Work out the finished part from the listing and answer in its coordinate system (mm). Round coordinates to 2 decimals unless told otherwise and drop trailing zeros. Order: outer loops, then holes, each group sorted by start corner. A loop starts at its lowest first (then second) coordinate and runs counter-clockwise, first axis right, second up. Notation, with made-up numbers: (-16, -6) - (6, -6) arc R32 cw to (6, 31) - close; hole circle Ø6 at (-25, -23). An arc over 180 degrees is marked (long way). Answer in a Markdown table with one row per item.
from build123d import *

# Parameters (mm, degrees)
SKETCH1_R                                        = 3.5
BODY_DEPTH                                       = 3.175
F_6_GIMBAL_CLEARANCE_HOLE_D                      = 3.7973
F_6_GIMBAL_CLEARANCE_HOLE_DEPTH                  = 12
F_6_GIMBAL_CLEARANCE_HOLE_TIP                    = 1.140824014
CSK_FOR_M2_5_FLAT_HEAD_MACHINE_SCREW_D           = 2.9
CSK_FOR_M2_5_FLAT_HEAD_MACHINE_SCREW_CSINK_D     = 5.5
CSK_FOR_M2_5_FLAT_HEAD_MACHINE_SCREW_CSINK_ANGLE = 90
F_6_CIRCULAR_CLEARANCE_HOLES_D                   = 3.7973
F_6_CIRCULAR_CLEARANCE_HOLES_DEPTH               = 12
F_6_CIRCULAR_CLEARANCE_HOLES_TIP                 = 1.140824014
MOTOR_START                                      = 1.82626
SKETCH1_3_R                                      = 5
MOTOR_COLLAR_RELIEF_DEPTH                        = 135.039371942
F_6_32_TAPPED_HOLE_D                             = 2.7051
F_6_32_TAPPED_HOLE_DEPTH                         = 180.4416
F_6_32_TAPPED_HOLE_TIP                           = 0.81269403
FILLET1_R                                        = 6.35


with BuildPart() as part:
    # Sketch1 → Body (new body)
    with BuildSketch(Plane.XY):
        with BuildLine():
            Line((-29.36875, 100.140279829), (-29.36875, 87.440279829))
            Line((-29.36875, 87.440279829), (0, 87.440279829))
            Line((0, 87.440279829), (19.184718186, 66.158495963))
            Line((19.184718186, 66.158495963), (39.064677756, 56.735799561))
            Line((39.064677756, 56.735799561), (54.483635505, 89.266642494))
            ThreePointArc((54.483635505, 89.266642494), (49.996218262, 103.531501135), (35.431784746, 100.140279829))
            Line((35.431784746, 100.140279829), (6.35, 100.140279829))
            Line((6.35, 100.140279829), (6.35, 117.602779829))
            ThreePointArc((6.35, 117.602779829), (0, 123.952779829), (-6.35, 117.602779829))
            Line((-6.35, 117.602779829), (-6.35, 100.140279829))
            Line((-6.35, 100.140279829), (-29.36875, 100.140279829))
        make_face()
        with Locations((44.54365572, 93.977990695)):
            Circle(SKETCH1_R, mode=Mode.SUBTRACT)
    extrude(amount=BODY_DEPTH)

    # #6 Gimbal Clearance Hole
    with Locations(Plane(origin=(0, 108.077779829, 0), x_dir=(-1, 0, 0), z_dir=(0, 0, -1))):
        with Locations((0, 0), (0, 11.1125)):
            Hole(F_6_GIMBAL_CLEARANCE_HOLE_D / 2, depth=F_6_GIMBAL_CLEARANCE_HOLE_DEPTH)
            with Locations((0, 0, -(F_6_GIMBAL_CLEARANCE_HOLE_DEPTH + F_6_GIMBAL_CLEARANCE_HOLE_TIP / 2))):  # 118° drill point
                Cone(0, F_6_GIMBAL_CLEARANCE_HOLE_D / 2, F_6_GIMBAL_CLEARANCE_HOLE_TIP, mode=Mode.SUBTRACT)

    # CSK for M2.5 Flat Head Machine Screw (through all)
    with Locations(Plane(origin=(50.605833546, 97.477990695, 0), x_dir=(-1, 0, 0), z_dir=(0, 0, -1))):
        with Locations((0, 0), (6.062177826, -10.5), (12.124355653, 0)):
            CounterSinkHole(CSK_FOR_M2_5_FLAT_HEAD_MACHINE_SCREW_D / 2, CSK_FOR_M2_5_FLAT_HEAD_MACHINE_SCREW_CSINK_D / 2, counter_sink_angle=CSK_FOR_M2_5_FLAT_HEAD_MACHINE_SCREW_CSINK_ANGLE)

    # #6 Circular Clearance Holes
    with Locations(Plane(origin=(-20.32, 93.790279829, 0), x_dir=(-1, 0, 0), z_dir=(0, 0, -1))):
        with Locations((0, 0), (-20.32, 0), (-40.64, 0)):
            Hole(F_6_CIRCULAR_CLEARANCE_HOLES_D / 2, depth=F_6_CIRCULAR_CLEARANCE_HOLES_DEPTH)
            with Locations((0, 0, -(F_6_CIRCULAR_CLEARANCE_HOLES_DEPTH + F_6_CIRCULAR_CLEARANCE_HOLES_TIP / 2))):  # 118° drill point
                Cone(0, F_6_CIRCULAR_CLEARANCE_HOLES_D / 2, F_6_CIRCULAR_CLEARANCE_HOLES_TIP, mode=Mode.SUBTRACT)

    # Sketch1<3> → Motor Collar Relief (cut, through all)
    with BuildSketch(Plane.XY.offset(MOTOR_START)):
        with Locations((44.54365572, 93.977990695)):
            Circle(SKETCH1_3_R)
    extrude(amount=MOTOR_COLLAR_RELIEF_DEPTH, mode=Mode.SUBTRACT)

    # #6-32 Tapped Hole
    with Locations(Plane(origin=(32.122828644, 67.772589444, 0), x_dir=(-1, 0, 0), z_dir=(0, 0, -1))):
        with Locations((0, 0)):
            Hole(F_6_32_TAPPED_HOLE_D / 2, depth=F_6_32_TAPPED_HOLE_DEPTH)
            with Locations((0, 0, -(F_6_32_TAPPED_HOLE_DEPTH + F_6_32_TAPPED_HOLE_TIP / 2))):  # 118° drill point
                Cone(0, F_6_32_TAPPED_HOLE_D / 2, F_6_32_TAPPED_HOLE_TIP, mode=Mode.SUBTRACT)

    # Fillet1
    fillet1_edges = [part.edges().sort_by_distance(p)[0] for p in [
        (0, 87.440279829, 1.5875),
        (-29.36875, 87.440279829, 1.5875),
        (-29.36875, 100.140279829, 1.5875),
        (-6.35, 100.140279829, 1.5875),
        (6.35, 100.140279829, 1.5875),
        (35.431784746, 100.140279829, 1.5875),
        (39.064677756, 56.735799561, 1.5875),
        (19.184718186, 66.158495963, 1.5875),
    ]]
    fillet(fillet1_edges, radius=FILLET1_R - 0.0001)  # a hair under: the kernel refuses the full size


solid = part.part
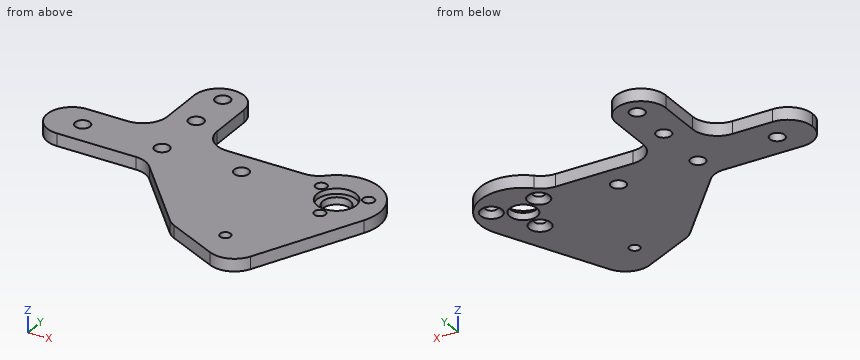
1) Find section D-D, the plane y = 115.5. Give the vertices of the cut face in (x, z) (3 decimals), then the cut area to 3 significant figures.
Filled in:
| item | result |
|---|---|
| outline | (-6.35, 0) - (6.35, 0) - (6.35, 3.175) - (-6.35, 3.175) - close |
| area | 40.3 mm^2 |
2) Find the intervals of material crossed by probe 1 along Y at (x, z) = (20.32, 0.7); probe 2 along Y at (x, z) = (0, 1.45); probe 3 along Y at (x, z) = (-23, 0.6), in increasing order. Write a range as from..to.
Filled in:
| item | result |
|---|---|
| probe 1 | y = 65.62..91.89, 95.69..100.14 |
| probe 2 | y = 86.78..91.89, 95.69..106.18, 109.98..117.29, 121.09..123.95 |
| probe 3 | y = 87.44..100.14 |
3) Find section C-C, the plane x = 0. Give the vertices of the cut face in (y, z) (3 decimals).
Filled in:
| item | result |
|---|---|
| outline | (86.777, 0) - (91.892, 0) - (91.892, 3.175) - (86.777, 3.175) - close; (95.689, 0) - (106.179, 0) - (106.179, 3.175) - (95.689, 3.175) - close; (109.976, 0) - (117.292, 0) - (117.292, 3.175) - (109.976, 3.175) - close; (121.089, 0) - (123.953, 0) - (123.953, 3.175) - (121.089, 3.175) - close |
4) Find section A-A, the plane x = -20.32. Give the vertices of the cut face in (y, z) (3 decimals).
Filled in:
| item | result |
|---|---|
| outline | (87.44, 0) - (91.892, 0) - (91.892, 3.175) - (87.44, 3.175) - close; (95.689, 0) - (100.14, 0) - (100.14, 3.175) - (95.689, 3.175) - close |
5) Each of these flat-tipped pins is pushed along its axis until it touches: pin 1 (4 mm diameter, centred on x = 50.61, y = 97.48, fed in from -Z); pin 2 (2.5 mm diameter, centred on x = 38.48, y = 97.48, fed in from -Z); pin 3 (3.5 mm diameter, centred on x = 44.54, y = 86.98, fed in from -Z); pin 4 (1.5 mm diameter, centred on y = 107.5, z = 1.5, fed in from +X). Where does it stop, or does it pass through?
Filled in:
| item | result |
|---|---|
| pin 1 | stops at z = 0.75 |
| pin 2 | passes through |
| pin 3 | stops at z = 1 |
| pin 4 | stops at x = 6.35 |
6) Find section B-B, the plane z = 2.65. Give the number of separate pieces and of enclosed holes in the cut face, then the cut area to 3 significant figures.
Filled in:
| item | result |
|---|---|
| separate pieces | 1 |
| enclosed holes | 10 |
| area | 2,190 mm^2 |
